The listing builds one solid part. Answer for the finished solid, in the listing's coordinates (mm). Give positions to 0.01 mm unless a question says otherwise; leave off trailing zeros. Loops run counter-clockwise (first coordinate to the right, second up) from the corner with the lowest first, then second, coordinate; pieces in that order, holes last. Notation, with made-up numbers: (-8.75, 26) - (24.25, 26) arc R22 ccw to (24.25, 32) - close; hole circle Ø5 at (52.25, 80.5). An arc over 180 degrees is marked (long way). Write each question's results on one line, items separated by ' | '.
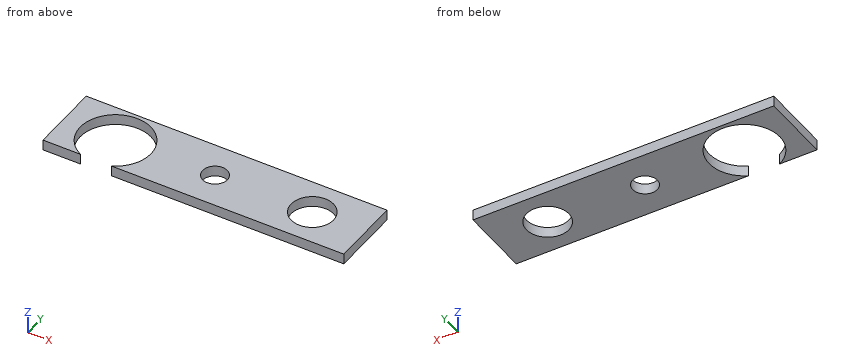
from build123d import *

# Parameters (mm, degrees)
SKETCH1_W           = 85
SKETCH1_H           = 20
BOSS_EXTRUDE1_DEPTH = 3
SKETCH2_R           = 3.5
SKETCH2_R_2         = 6
SKETCH2_R_3         = 10
CUT_EXTRUDE1_DEPTH  = 4


with BuildPart() as part:
    # Sketch1 → Boss-Extrude1 (new body)
    with BuildSketch(Plane.XY):
        with Locations((42.5, 10)):
            Rectangle(SKETCH1_W, SKETCH1_H)
    extrude(amount=BOSS_EXTRUDE1_DEPTH)

    # Sketch2 → Cut-Extrude1 (cut, through all)
    with BuildSketch(Plane.XY.offset(3)):
        with Locations((42.5, 10)):
            Circle(SKETCH2_R)
        with Locations((70, 10)):
            Circle(SKETCH2_R_2)
        with Locations((15, 9)):
            Circle(SKETCH2_R_3)
    extrude(amount=-CUT_EXTRUDE1_DEPTH, mode=Mode.SUBTRACT)


solid = part.part
Item 1: A cutting plane is placed at A-A, the plane x = 9. Determine the outline of the cut face in (y, z).
Values found:
outline: (0, 0) - (1, 0) - (1, 3) - (0, 3) - close; (17, 0) - (20, 0) - (20, 3) - (17, 3) - close
Item 2: A cutting plane is placed at B-B, the plane z = 0.65. Determine the outline of the cut face in (x, y).
Values found:
outline: (0, 0) - (10.64, 0) arc R10 cw (long way) to (19.36, 0) - (85, 0) - (85, 20) - (0, 20) - close; hole circle Ø7 at (42.5, 10); hole circle Ø12 at (70, 10)
Item 3: A cutting plane is placed at D-D, the plane x = 42.5. Determine the outline of the cut face in (y, z), plus the area to 3 significant figures.
Values found:
outline: (0, 0) - (6.5, 0) - (6.5, 3) - (0, 3) - close; (13.5, 0) - (20, 0) - (20, 3) - (13.5, 3) - close | area: 39.0 mm²
Item 4: A cutting plane is placed at C-C, the plane y = 12.25. Determine the outline of the cut face in (x, z).
Values found:
outline: (0, 0) - (5.54, 0) - (5.54, 3) - (0, 3) - close; (24.46, 0) - (39.82, 0) - (39.82, 3) - (24.46, 3) - close; (45.18, 0) - (64.44, 0) - (64.44, 3) - (45.18, 3) - close; (75.56, 0) - (85, 0) - (85, 3) - (75.56, 3) - close
Item 5: Find the intervals of material crossed by line 1 along Y through (x, z) = (70, 2.35); line 2 along X through (y, z) = (5.25, 0.4); line 3 along X through (y, z) = (3.5, 0.5), in increasing order. Write a range as [from, to].
Values found:
line 1: y = [0, 4], [16, 20] | line 2: x = [0, 5.73], [24.27, 66.33], [73.67, 85] | line 3: x = [0, 6.65], [23.35, 85]
